```python
from build123d import *

# Parameters (mm, degrees)
F0_R     = 2
F1_DEPTH = 10
F2_W     = 12
F2_H     = 20
F3_DEPTH = 2


with BuildPart() as f1:
    # F0 (on Top) → F1 (new body, symmetric)
    with BuildSketch(Plane.XY):
        Circle(F0_R)
    extrude(amount=F1_DEPTH, both=True)

    # F2 (on Front) → F3 (join, symmetric)
    with BuildSketch(Plane.XZ):
        with Locations((6, -0.047689)):
            Rectangle(F2_W, F2_H)
    extrude(amount=F3_DEPTH, both=True)


solid = f1.part
```
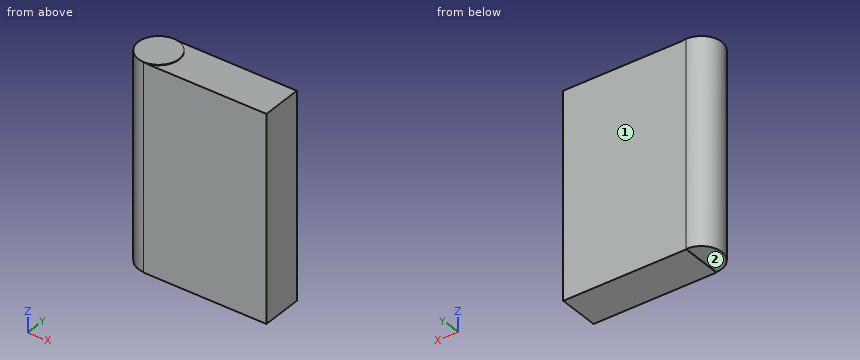
CAD build for the part. Positions are in the model's coordinates, mm. Face numbers are marked on the shaded views. A direction names the side the tool comes from. Round coordinates to 2 decimals unless told otherwise and drop trailing zeros. Order: outer loops, then holes, each group sorted by start corner. A loop starts at its lowest first (then second) coordinate and runs counter-clockwise, first axis right, second up. Notation, with made-up numbers: (74.25, 80.5) - (108.25, 80.5) arc R12 cw to (108.25, 93.5) - close; hole circle Ø9 at (31.5, -16). An arc over 180 degrees is marked (long way). Answer as CSV lines item,"result". Start each with the question number.
1. Saw through at A-A, the plane z = 0.75. Write the cut outline in (x, y), and give its area (3 significant figures).
2. Saw through at C-C, the plane x = -0.75. Write the cut outline in (y, z), and give its area (3 significant figures).
3. Pin check, flat tip, straight feed: pin 1 (0.6 mm diameter, centred on x = -1.5, y = 1, fed in from -Z). Stop position of the tip, or through.
4. Tool access for the marked faces 1 and 2: list every direction of +Z, -Z, +X, -X, +Y, -Y with a clear straight run to the whole face (end or side of a thin tool).
5. Drill centre lines: L1, parallel to Z at x = 11, y = -1.4; L2, parallel to X at y = 0.3, z = 2.25; L3, parallel to X at y = 1.65, z = 9. Where is each one in solid material? Low to high. Write a range as [from, to].
6. Saw through at B-B, the plane y = 1.7. Write the cut outline in (x, z).
Model answer:
1,outline,"(0, -2) - (12, -2) - (12, 2) - (0, 2) arc R2 ccw to start"
1,area,"54.3 mm²"
2,outline,"(-1.85, -10) - (1.85, -10) - (1.85, 10) - (-1.85, 10) - close"
2,area,"74.2 mm²"
3,pin 1,"stops at z = -10"
4,face 1,"+Z, -Z, +X, -X, +Y"
4,face 2,"-Z, -X, +Y, -Y"
5,L1,"z = [-10.05, 9.95]"
5,L2,"x = [-1.98, 12]"
5,L3,"x = [-1.13, 12]"
6,outline,"(-1.05, -10) - (0, -10) - (0, -10.05) - (12, -10.05) - (12, 9.95) - (1.05, 9.95) - (1.05, 10) - (-1.05, 10) - close"
